Can you work these out from the model? Positions are in its coordinate system, mm. Face numbers are marked on the shaded views. A direction names the side the tool comes from. Give positions to 0.01 mm unless a question says otherwise; leave off trailing zeros. Order: outer loops, then holes, each group sorted by start corner. A loop starts at its lowest first (then second) coordinate and runs counter-clockwise, first axis right, second up.
Item 1: I want a section at D-D, the plane y = -96.5. Write out the boundary of the cut face in (x, z), then the cut area to 3 significant figures.
Item 2: I want a section at C-C, the plane x = 66.5. Write out the boundary of the cut face in (y, z), then the cut area to 3 significant figures.
Item 3: I'm going to push flat-ended pins straight in: pin 1 Ø8 at (x, z) = (-8, 7.5) entering from -Y; pin 2 Ø9 at (y, z) = (-142.5, -15) entering from +X; pin 3 Ø1 at (y, z) = (49, -11.5) entering from -X. Where does each tip first touch, or does it pass through?
Item 4: If we mould it in two halves opening along Y, with no side actions, what happens to the marked faces 6, 7 and 8? For each: +Y half, -Y half, draft (parallel to the pull), parting line (faces both ways), or undercut.
Item 5: I want a section at A-A, the plane z = 71. Write out the boundary of the cut face in (x, y), then the cut area to 3 significant figures.
Item 6: If I drill on line 1 along X through (y, z) = (97.5, 28.5); line 2 along Y through (x, z) = (-51.5, 16); line 3 along Z through (x, y) = (-2.5, 69.5), over which ranges is the centre line in solid material (lowest first)?
Item 7: Which directions (+Z, -Z, +X, -X, +Y, -Y) give clear straight access to the entire face, cutting with the end or side of a thin tool? Please do the marked faces 1, 2, 3, 4 and 5.
Item 8: I want a section at B-B, the plane z = -7. Write out the boundary of the cut face in (x, y), then the cut area to 3 significant figures.
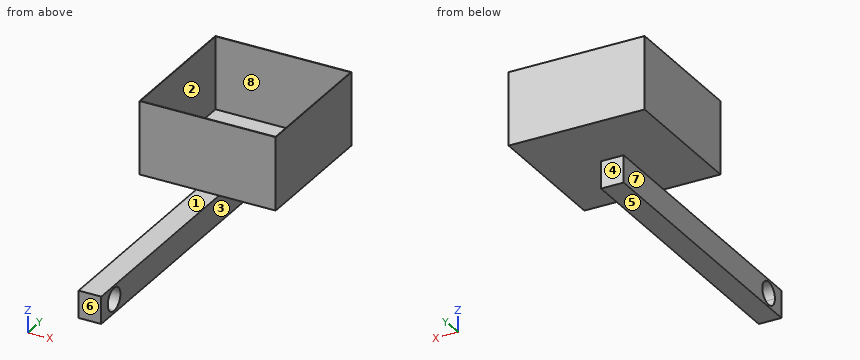
```python
from build123d import *

# Parameters (mm, degrees)
F0_W     = 0.5
F0_H     = 149
F1_DEPTH = 80
F2_W     = 150
F2_H     = 150
F3_DEPTH = 0.5
F5_DEPTH = 30
F7_DEPTH = 87.501
F9_DEPTH = 87.501


with BuildPart() as f1:
    # F0 (on Top) → F1 (new body)
    with BuildSketch(Plane.XY):
        Polygon((88.1122936055, 138.4297020262), (-61.8877063945, 138.4297020262), (-61.8877063945, 137.9297020262), (-61.3877063945, 137.9297020262), (87.6122936055, 137.9297020262), (88.1122936055, 137.9297020262), align=None)
        with Locations((-61.6377063945, 63.4297020262)):
            Rectangle(F0_W, F0_H)
        with Locations((87.8622936055, 63.4297020262)):
            Rectangle(F0_W, F0_H)
        Polygon((-61.3877063945, -11.0702979738), (-61.8877063945, -11.0702979738), (-61.8877063945, -11.5702979738), (88.1122936055, -11.5702979738), (88.1122936055, -11.0702979738), (87.6122936055, -11.0702979738), align=None)
    extrude(amount=F1_DEPTH)

    # F2 (on face) → F3 (join)
    with BuildSketch(Plane(origin=(0, 0, 0), x_dir=(1, 0, 0), z_dir=(0, 0, -1))):
        with Locations((13.1122936055, -63.4297020262)):
            Rectangle(F2_W, F2_H)
    extrude(amount=F3_DEPTH)

    # F4 (on face) → F5 (join)
    with BuildSketch(Plane(origin=(0, 0, -0.5), x_dir=(1, 0, 0), z_dir=(0, 0, -1))):
        Polygon((0.6122936055, -67.6260187756), (25.6122936055, -67.6260187756), (25.6122936055, 11.5702979738), (25.6122936055, 244.7964921594), (0.6122936055, 244.7964921594), (0.6122936055, 11.5702979738), align=None)
    extrude(amount=F5_DEPTH)

    # F6 (on face) → F7 (cut, through all)
    with BuildSketch(Plane.YZ.offset(25.6122936055)):
        with BuildLine():
            Line((85.952706635, -16.575855797), (85.952706635, -14.424144203))
            ThreePointArc((85.952706635, -14.424144203), (84.876850838, -15.5), (85.952706635, -16.575855797))
        make_face()
        with BuildLine():
            ThreePointArc((87.028562432, -15.5), (86.7134515646, -14.7392550704), (85.952706635, -14.424144203))
            Line((85.952706635, -14.424144203), (85.952706635, -16.575855797))
            ThreePointArc((85.952706635, -16.575855797), (86.7134515646, -16.2607449296), (87.028562432, -15.5))
        make_face()
    extrude(amount=-F7_DEPTH, mode=Mode.SUBTRACT)

    # F8 (on face) → F9 (cut, through all)
    with BuildSketch(Plane(origin=(0.6122936055, 0, 0), x_dir=(0, -1, 0), z_dir=(-1, 0, 0))):
        with BuildLine():
            ThreePointArc((231.8976938725, -15.5), (228.2365286373, -6.6611652352), (219.3976938725, -3))
            Line((219.3976938725, -3), (219.3976938725, -28))
            ThreePointArc((219.3976938725, -28), (228.2365286373, -24.3388347648), (231.8976938725, -15.5))
        make_face()
        with BuildLine():
            Line((219.3976938725, -28), (219.3976938725, -3))
            ThreePointArc((219.3976938725, -3), (206.8976938725, -15.5), (219.3976938725, -28))
        make_face()
    extrude(amount=-F9_DEPTH, mode=Mode.SUBTRACT)


solid = f1.part
```
Results list:
1. outline: (0.61, -30.5) - (25.61, -30.5) - (25.61, -0.5) - (0.61, -0.5) - close
1. area: 750 mm2
2. outline: (-11.57, -0.5) - (138.43, -0.5) - (138.43, 80) - (137.93, 80) - (137.93, 0) - (-11.07, 0) - (-11.07, 80) - (-11.57, 80) - close
2. area: 155 mm2
3. pin 1: stops at y = -11.57
3. pin 2: stops at x = 25.61
3. pin 3: stops at x = 0.61
4. face 6: -Y half
4. face 7: draft
4. face 8: undercut
5. outline: (-61.89, -11.57) - (88.11, -11.57) - (88.11, 138.43) - (-61.89, 138.43) - close; hole (-61.39, -11.07) - (87.61, -11.07) - (87.61, 137.93) - (-61.39, 137.93) - close
5. area: 299 mm2
6. line 1: x = -61.89 to -61.39, 87.61 to 88.11
6. line 2: y = -11.57 to -11.07, 137.93 to 138.43
6. line 3: z = -0.5 to 0
7. face 1: +Z, +X, -X, -Y
7. face 2: +Z
7. face 3: -Z, +X, +Y, -Y
7. face 4: -Z, +X, -X, +Y
7. face 5: -Z, +X, -X, +Y, -Y
8. outline: (0.61, -244.8) - (25.61, -244.8) - (25.61, -228.56) - (0.61, -228.56) - close; (0.61, -210.23) - (25.61, -210.23) - (25.61, 67.63) - (0.61, 67.63) - close
8. area: 7,350 mm2
